Input: part model. Units: mm. Frame: model coordinates. A direction names the side the tool comes from. Coordinates: 2 decimals unless noted, no trailing zeros. Loops run counter-clockwise (first coordinate to the right, second up) from the corner with the lowest first, then second, coordinate; pieces in that order, holes last. Notation, with made-up numbers: (44, -8.75) - (66, -8.75) arc R15 cw to (66, 6.25) - close; hole circle Ø1 at (53.25, 57). An arc over 180 degrees is marked (long way). Use one line per item in the form item = value.
from build123d import *

# Parameters (mm, degrees)
F0_W      = 215.9
F0_H      = 44.45
F1_DEPTH  = 76.2
F2_T      = -5.08
F3_W      = 6.35
F3_H      = 76.2
F5_DEPTH  = 12.7
F4_W      = 6.35
F4_H      = 76.2
F6_DEPTH  = 12.7
F8_W      = 6.35
F8_H      = 50.8
F9_DEPTH  = 12.7
F10_W     = 6.35
F10_H     = 50.8
F11_DEPTH = 12.7
F12_W     = 6.35
F12_H     = 50.8
F13_DEPTH = 12.7
F14_W     = 6.35
F14_H     = 50.8
F15_DEPTH = 12.7
F16_W     = 152.4
F16_H     = 46.080392
F17_DEPTH = 5.08
F7_R      = 6
F18_DEPTH = 5.08
F20_W     = 1.905
F20_H     = 6.35
F19_W     = 1.905
F19_H     = 6.35
F21_DEPTH = 25.4


with BuildPart() as f1:
    # F0 (on Top) → F1 (new body)
    with BuildSketch(Plane.XY):
        with Locations((-2.774038, 0)):
            Rectangle(F0_W, F0_H)
    extrude(amount=F1_DEPTH)

    # F2
    f2_openings = [f1.faces().sort_by_distance(p)[0] for p in [
        (-2.774038, 0, 0),
    ]]
    offset(amount=F2_T, openings=f2_openings)

    # F3 (on face) → F5 (join)
    with BuildSketch(Plane.XZ.offset(22.225)):
        with Locations((-107.549038, 38.1)):
            Rectangle(F3_W, F3_H)
        with Locations((102.000962, 38.1)):
            Rectangle(F3_W, F3_H)
    extrude(amount=F5_DEPTH)

    # F4 (on face) → F6 (join)
    with BuildSketch(Plane(origin=(0, 22.225, 0), x_dir=(-1, 0, 0), z_dir=(0, 1, 0))):
        with Locations((-102.000962, 38.1)):
            Rectangle(F4_W, F4_H)
        with Locations((107.549038, 38.1)):
            Rectangle(F4_W, F4_H)
    extrude(amount=F6_DEPTH)

    # F8 (on face) → F9 (join)
    with BuildSketch(Plane.YZ.offset(-104.374038)):
        Polygon((-28.575, 76.2), (-34.925, 76.2), (-34.925, 0), (-28.575, 0), (-28.575, 50.8), align=None)
        with Locations((-25.4, 25.4)):
            Rectangle(F8_W, F8_H)
    extrude(amount=F9_DEPTH)

    # F10 (on face) → F11 (join)
    with BuildSketch(Plane(origin=(98.825962, 0, 0), x_dir=(0, -1, 0), z_dir=(-1, 0, 0))):
        Polygon((34.925, 0), (34.925, 76.2), (28.575, 76.2), (28.575, 50.8), (28.575, 0), align=None)
        with Locations((25.4, 25.4)):
            Rectangle(F10_W, F10_H)
    extrude(amount=F11_DEPTH)

    # F12 (on face) → F13 (join)
    with BuildSketch(Plane(origin=(98.825962, 0, 0), x_dir=(0, -1, 0), z_dir=(-1, 0, 0))):
        Polygon((-34.925, 76.2), (-34.925, 0), (-28.575, 0), (-28.575, 50.8), (-28.575, 76.2), align=None)
        with Locations((-25.4, 25.4)):
            Rectangle(F12_W, F12_H)
    extrude(amount=F13_DEPTH)

    # F14 (on face) → F15 (join)
    with BuildSketch(Plane.YZ.offset(-104.374038)):
        Polygon((34.925, 0), (34.925, 76.2), (28.575, 76.2), (28.575, 50.8), (28.575, 0), align=None)
        with Locations((25.4, 25.4)):
            Rectangle(F14_W, F14_H)
    extrude(amount=F15_DEPTH)

    # F16 (on face) → F17 (cut)
    with BuildSketch(Plane(origin=(0, 22.225, 0), x_dir=(-1, 0, 0), z_dir=(0, 1, 0))):
        with Locations((2.774038, 23.040196)):
            Rectangle(F16_W, F16_H)
    extrude(amount=-F17_DEPTH, mode=Mode.SUBTRACT)

    # F7 (on face) → F18 (cut)
    with BuildSketch(Plane.XY.offset(76.2)):
        with Locations((67.075962, -6.731)):
            Circle(F7_R)
        with Locations((32.150962, -6.731)):
            Circle(F7_R)
        with Locations((-2.774038, -6.731)):
            Circle(F7_R)
        with Locations((-37.699038, -6.731)):
            Circle(F7_R)
        with Locations((-72.624038, -6.731)):
            Circle(F7_R)
    extrude(amount=-F18_DEPTH, mode=Mode.SUBTRACT)

    # F20 (on face) + F19 (on face) → F21 (join)
    with BuildSketch(Plane.XY.offset(50.8)):
        with Locations((-103.421538, 25.4)):
            Rectangle(F20_W, F20_H)
    with BuildSketch(Plane.XY.offset(50.8)):
        with Locations((97.873462, 25.4)):
            Rectangle(F19_W, F19_H)
    extrude(amount=F21_DEPTH)


solid = f1.part
Q1. Ray query, line 1 along Y through (x, z) = (-13.5, 58.5) (3 decimals); line 2 along X through (y, z) = (-25.5, 66.5); line 3 along X through (y, z) = (-12, 44). Return the intervals inside material, ascending. Write a range as [from, to].
Check values:
line_1 = [-22.225, -17.145], [17.145, 22.225]
line_2 = [-110.72, -104.37], [98.83, 105.18]
line_3 = [-110.72, -105.64], [100.1, 105.18]
Q2. Cut plane C-C, the plane x = -23.5. Return loops of the section in (y, z) (3 decimals).
Check values:
outline = (-22.225, 0) - (-17.145, 0) - (-17.145, 71.12) - (17.145, 71.12) - (17.145, 46.08) - (22.225, 46.08) - (22.225, 76.2) - (-22.225, 76.2) - close
Q3. Pull-direction query (X, two-part tool) for faces 1 (the flat face through (96.921, 25, 63)), 2 (the flat face through (-3, -18, 0)); classes: pulls with the +X half, pulls with the -X half, needs draft (parallel to the pull), parting line crosses it, or undercut.
Check values:
face_1 = undercut
face_2 = needs draft
Q4. Cut plane A-A, the plane z = 63. Return loops of the section in (x, y) (3 decimals).
Check values:
outline = (-110.724, -34.925) - (-91.674, -34.925) - (-91.674, -28.575) - (-104.374, -28.575) - (-104.374, -22.225) - (98.826, -22.225) - (98.826, -28.575) - (86.126, -28.575) - (86.126, -34.925) - (105.176, -34.925) - (105.176, 34.925) - (86.126, 34.925) - (86.126, 28.575) - (96.921, 28.575) - (96.921, 22.225) - (-102.469, 22.225) - (-102.469, 28.575) - (-91.674, 28.575) - (-91.674, 34.925) - (-110.724, 34.925) - close; hole (-105.644, -17.145) - (100.096, -17.145) - (100.096, 17.145) - (-105.644, 17.145) - close
Q5. Cut plane B-B, the plane y = -15. Return loops of the section in (x, z), then the cut area to 3 significant figures.
Check values:
outline = (-110.72, 0) - (-105.64, 0) - (-105.64, 71.12) - (100.1, 71.12) - (100.1, 0) - (105.18, 0) - (105.18, 76.2) - (-110.72, 76.2) - close
area = 1,820 mm²
Q6. Set-up query: faces 3 (the flat face through (-4, 17.145, 51)), 4 (the flat face through (-78.974, 20, 23)), 5 (the flat face through (-102.469, 25, 63)), 6 (the flat face through (-91.674, -29, 30)). Return all of +Z, -Z, +X, -X, +Y, -Y with unobstructed straight access to the full face (end or side cutting, diameter ignored); none if empty.
Check values:
face_3 = -Z
face_4 = -Z, +Y
face_5 = +Z
face_6 = +Z, -Z, -Y
Q7. Cut plane D-D, the plane z = 14.5. Return loops of the section in (x, y) (3 decimals).
Check values:
outline = (-110.724, -34.925) - (-91.674, -34.925) - (-91.674, -22.225) - (86.126, -22.225) - (86.126, -34.925) - (105.176, -34.925) - (105.176, 34.925) - (86.126, 34.925) - (86.126, 22.225) - (73.426, 22.225) - (73.426, 17.145) - (100.096, 17.145) - (100.096, -17.145) - (-105.644, -17.145) - (-105.644, 17.145) - (-78.974, 17.145) - (-78.974, 22.225) - (-91.674, 22.225) - (-91.674, 34.925) - (-110.724, 34.925) - close
Q8. First-contact query: P1, Ø3, axis at x = -95.5, y = -24.5, coming from the +Z side; P2, Ø11, axis at x = -2.77, y = -6.73, coming from the -Z side; P3, Ø21.5, axis at x = -1.5, z = 43.5, coming from the -Y side (3 decimals); P4, Ø1, axis at x = 74, z = 8, coming from the +Y side (3 decimals). Flat tips, straight axial feed; report the tip coordinate or a pass-through.
Check values:
P1 = 50.8
P2 = through
P3 = -22.225
P4 = 22.225
